The model under review builds one solid part; all positions refer to its coordinate system, in mm. Face numbers are marked on the shaded views. Give positions to 0.01 mm unless a question says otherwise; leave off trailing zeros. Order: outer loops, then holes, each group sorted by start corner. A loop starts at its lowest first (then second) coordinate and runs counter-clockwise, first axis right, second up.
```python
from build123d import *

# Parameters (mm, degrees)
F1_DEPTH = 120
F2_R     = 6
F3_DEPTH = 10
F4_R     = 5
F5_DEPTH = 423.023222


with BuildPart() as f1:
    # F0 (on Front) → F1 (new body)
    with BuildSketch(Plane.XZ):
        Polygon((-5, 50), (-5, 0), (5, 0), (5, 50), (50, 50), (50, 60), (-50, 60), (-50, 50), align=None)
    extrude(amount=F1_DEPTH)

    # F2 (on face) → F3 (join)
    with BuildSketch(Plane.YZ.offset(5)):
        Polygon((-29.358222, 20), (-60, 45.711504), (-381.393805, -337.310717), (-350.752027, -363.022222), align=None)
        with Locations((-327.505659, -304.203803)):
            Circle(F2_R, mode=Mode.SUBTRACT)
        with Locations((-295.366279, -265.901581)):
            Circle(F2_R, mode=Mode.SUBTRACT)
        with Locations((-263.226898, -227.599358)):
            Circle(F2_R, mode=Mode.SUBTRACT)
        with Locations((-231.087518, -189.297136)):
            Circle(F2_R, mode=Mode.SUBTRACT)
        with Locations((-198.631472, -151.262874)):
            Circle(F2_R, mode=Mode.SUBTRACT)
        with Locations((-60, 20)):
            Circle(F2_R, mode=Mode.SUBTRACT)
    extrude(amount=F3_DEPTH)

    # F4 (on face) → F5 (cut, through all)
    with BuildSketch(Plane.XY.offset(60)):
        with Locations((-32.022849, -10)):
            Circle(F4_R)
        with Locations((-32.022849, -60)):
            Circle(F4_R)
        with Locations((-32.022849, -110)):
            Circle(F4_R)
        with Locations((32.022849, -110)):
            Circle(F4_R)
        with Locations((32.022849, -60)):
            Circle(F4_R)
        with Locations((32.022849, -10)):
            Circle(F4_R)
    extrude(amount=-F5_DEPTH, mode=Mode.SUBTRACT)


solid = f1.part
```
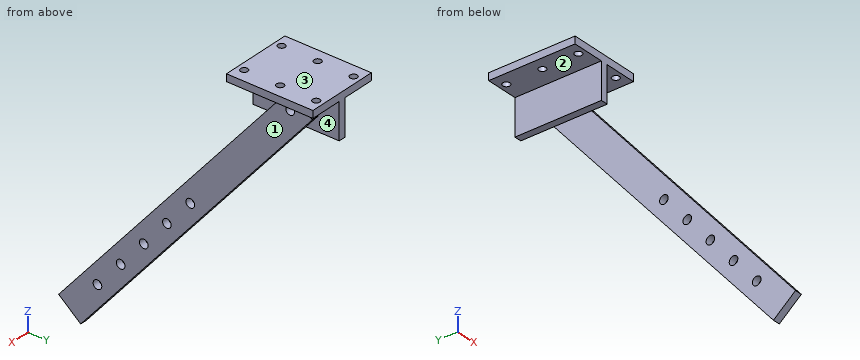
Item 1: Take a section at D-D (z = -202). Give the boundary of the cut face in (x, y), and give its area (3 significant figures).
Values found:
outline: (5, -267.85) - (15, -267.85) - (15, -215.64) - (5, -215.64) - close
area: 522 mm2
Item 2: For line 1 (Z direction, x = 32, y = -19); line 2 (X direction, y = -214.5, z = -167); line 3 (Y direction, x = 7, z = 15.5), list the stretches that pass through material, from the lowest coordinate up.
Values found:
line 1: z = 50 to 60
line 2: x = 5 to 15
line 3: y = -85.35 to -63.97, -56.03 to -33.13
Item 3: Clearance check with flat-ended pins moving along their axes: pin 1 Ø14 at (y, z) = (-60, 20) entering from -X; pin 2 Ø19 at (y, z) = (-231.09, -189.3) entering from +X; pin 3 Ø13 at (x, y) = (32.02, -110) entering from -Z; pin 4 Ø8 at (x, y) = (32.02, -10) entering from -Z. State where each tip first meets the part, or that it passes through.
Values found:
pin 1: stops at x = -5
pin 2: stops at x = 15
pin 3: stops at z = 50
pin 4: passes through
Item 4: Take a section at A-A (y = -10). Give the boundary of the cut face in (x, z), and give its area (3 significant figures).
Values found:
outline: (-50, 50) - (-37.02, 50) - (-37.02, 60) - (-50, 60) - close; (-27.02, 50) - (-5, 50) - (-5, 0) - (5, 0) - (5, 50) - (27.02, 50) - (27.02, 60) - (-27.02, 60) - close; (37.02, 50) - (50, 50) - (50, 60) - (37.02, 60) - close
area: 1,300 mm2
Item 5: Draft analysis for pull direction Z (two halves, no side actions). For the marked faces 1, 2, 3 and 4, state which applies: released by +Z, released by -Z, zero draft, split by the parting line, or undercut.
Values found:
face 1: zero draft
face 2: released by -Z
face 3: released by +Z
face 4: undercut
Item 6: Take a section at C-C (x = -11). Give the boundary of the cut face in (y, z), and give its area (3 significant figures).
Values found:
outline: (-120, 50) - (0, 50) - (0, 60) - (-120, 60) - close
area: 1,200 mm2
Item 7: Take a section at B-B (y = -110). Give the boundary of the cut face in (x, z).
Values found:
outline: (-50, 50) - (-37.02, 50) - (-37.02, 60) - (-50, 60) - close; (-27.02, 50) - (-5, 50) - (-5, 0) - (5, 0) - (5, 50) - (27.02, 50) - (27.02, 60) - (-27.02, 60) - close; (5, -76.11) - (15, -76.11) - (15, -13.88) - (5, -13.88) - close; (37.02, 50) - (50, 50) - (50, 60) - (37.02, 60) - close
